Model file for the job. Use its own axes, mm. Round coordinates to 2 decimals unless told otherwise and drop trailing zeros. Order: outer loops, then holes, each group sorted by start corner. A loop starts at its lowest first (then second) coordinate and runs counter-clockwise, first axis right, second up. Notation, with made-up numbers: (-38, 77.25) -> (-1, 77.25) arc R23 ccw to (-1, 112.25) -> close; hole circle Ø3 at (-24, 10.25). An arc over 180 degrees is marked (long way). Use CSV: the item, a comma, the result in double quotes.
```python
from build123d import *

# Parameters (mm, degrees)
F0_R     = 13.75969411
F1_DEPTH = 100
F3_DEPTH = 100.001
F4_SIZE2 = 56.1456900142
F4_SIZE  = 9.9
F5_R     = 261.7912381488


# Not quite as in the source:
# - a fillet or chamfer that OpenCascade refuses, or shapes differently, is made with other operations: its cross-section is extruded or revolved along the edge and cut away or added


with BuildPart() as f1:
    # F0 (on Top) → F1 (new body)
    with BuildSketch(Plane.XY):
        with Locations((-55.1216676831, -44.3151853979)):
            Circle(F0_R)
    extrude(amount=F1_DEPTH)

    # F2: fillet of radius 12.0710678119 on 1 edges, made by hand

    # F2_s1 → F2_t2 (revolve, cut)
    with BuildSketch(Plane.XZ.offset(44.3151853979)):
        with BuildLine():
            add(Edge.make_bspline(
                [(-41.3619735731, 12.0710678119), (-41.3619735731, 0), (-53.433041385, 0)],
                knots=[0, 0, 0, 1, 1, 1], degree=2, weights=[1, 0.4285714286, 1]))
            Line((-53.433041385, 0), (-41.3619735731, 0))
            Line((-41.3619735731, 0), (-41.3619735731, 12.0710678119))
        make_face()
    revolve(axis=Axis((-55.1216676831, -44.3151853979, 0), (0, 0, 1)), mode=Mode.SUBTRACT)

    # F3 (cut, through all): a face of the model
    f3_faces = [f1.faces().sort_by_distance(p)[0] for p in [
        (-55.1216676831, -44.3151853979, 0),
    ]]
    extrude(f3_faces, amount=-F3_DEPTH, mode=Mode.SUBTRACT)

    # F4
    f4_edges = [f1.edges().sort_by_distance(p)[0] for p in [
        (-68.881362, -44.315185, 100),
    ]]
    f4_side = f1.faces().sort_by_distance((-68.492179, -44.315185, 100))[0]
    chamfer(f4_edges, length=F4_SIZE, length2=F4_SIZE2, reference=f4_side)

    # F5
    f5_edges = [f1.edges().sort_by_distance(p)[0] for p in [
        (-68.881362, -44.315185, 43.85431),
    ]]
    fillet(f5_edges, radius=F5_R)


solid = f1.part
```
Q1. Probe line 1 along X through (y, z) = (-44, 56.5); line 2 along X through (y, z) = (-45.25, 13.5); line 3 along Y through (x, z) = (-56.25, 6.5). List the from-to ranges inside material, lowest first.
From the geometry:
line 1,"x = -66.45 to -56.78, -53.46 to -43.79"
line 2,"x = -68.85 to -56.53, -53.72 to -41.39"
line 3,"y = -55.74 to -45.57, -43.06 to -32.89"
Q2. Mould opens along X. For faces 1 (the cylindrical face through (-42, -40.18, 16.45)), 2 (the flat face through (-54, -46, 100)), 3 (the cylindrical face through (-56.81, -44.24, 49.3)) say: +X half, -X half, draft (parallel to the pull), parting line (faces both ways), or undercut.
From the geometry:
face 1,"parting line"
face 2,"draft"
face 3,"undercut"
Q3. Cut at A-A (z = 83.5). Give the cut face in (x, y), plus the area to 3 significant figures.
From the geometry:
outline,"circle Ø13.54 at (-55.12, -44.32); hole circle Ø3.38 at (-55.12, -44.32)"
area,"135 mm²"
Q4. Cut at B-B (z = 14.5). Give the cut face in (x, y), plus the area to 3 significant figures.
From the geometry:
outline,"circle Ø27.52 at (-55.12, -44.32); hole circle Ø3.38 at (-55.12, -44.32)"
area,"586 mm²"
Q5. Pin check, flat tips, straight feed: pin 1 (2 mm diameter, centred on y = -39.5, z = 85.5, fed in from +X); pin 2 (12 mm diameter, centred on x = -46.5, y = -50.5, fed in from -Z); pin 3 (3 mm diameter, centred on y = -48, z = 62, fed in from +X). Stop position of each tip, or through.
From the geometry:
pin 1,"stops at x = -49.93"
pin 2,"stops at z = 0.72"
pin 3,"stops at x = -44.75"
